from build123d import *

# Parameters (mm, degrees)
MODEL_R                  = 1.8
RESSALTO_EXTRUS_O1_DEPTH = 6


with BuildPart() as part:
    # Model → Ressalto-extrusão1 (new body)
    with BuildSketch(Plane.XY):
        Polygon((65.723755116, 35.074422304), (65.623854693, 35.315603259), (65.46493607, 35.52271004), (65.257829289, 35.681628662), (65.016648334, 35.781529085), (64.757829289, 35.815603259), (50.157829289, 35.815603259), (50.157829289, 33.103327835), (43.557829289, 33.103327835), (43.557829289, 56.603327835), (50.157829289, 56.603327835), (50.157829289, 50.820791423), (59.157829289, 50.820791423), (59.157829289, 56.103327835), (64.757829289, 56.103327835), (65.016648334, 56.137402008), (65.257829289, 56.237302431), (65.46493607, 56.396221053), (65.623854693, 56.603327835), (65.723755116, 56.844508789), (65.757829289, 57.103327835), (65.757829289, 61.703327835), (65.723755116, 61.96214688), (65.623854693, 62.203327835), (65.46493607, 62.410434616), (65.257829289, 62.569353238), (65.016648334, 62.669253661), (64.757829289, 62.703327835), (59.157829289, 62.703327835), (59.157829289, 67.703327835), (35.557829289, 67.703327835), (35.557829289, 59.703327835), (29.957829289, 59.703327835), (29.699010244, 59.669253661), (29.457829289, 59.569353238), (29.250722508, 59.410434616), (29.091803885, 59.203327835), (28.991903463, 58.96214688), (28.957829289, 58.703327835), (28.957829289, 50.703327835), (28.991903463, 50.444508789), (29.091803885, 50.203327835), (29.250722508, 49.996221053), (29.457829289, 49.837302431), (29.699010244, 49.737402008), (29.957829289, 49.703327835), (35.557829289, 49.703327835), (35.557829289, 30.703327835), (29.957829289, 30.703327835), (29.699010244, 30.669253661), (29.457829289, 30.569353238), (29.250722508, 30.410434616), (29.091803885, 30.203327835), (28.991903463, 29.96214688), (28.957829289, 29.703327835), (28.957829289, 21.703327835), (28.991903463, 21.444508789), (29.091803885, 21.203327835), (29.250722508, 20.996221053), (29.457829289, 20.837302431), (29.699010244, 20.737402008), (29.957829289, 20.703327835), (35.557829289, 20.703327835), (35.557829289, 12.703327835), (59.157829289, 12.703327835), (59.157829289, 20.903327835), (64.757829289, 20.903327835), (65.016648334, 20.937402008), (65.257829289, 21.037302431), (65.46493607, 21.196221053), (65.623854693, 21.403327835), (65.723755116, 21.644508789), (65.757829289, 21.903327835), (65.757829289, 34.815603259), align=None)
        with Locations((54.657829289, 63.703327835)):
            Circle(MODEL_R, mode=Mode.SUBTRACT)
        with Locations((54.657829289, 16.703327835)):
            Circle(MODEL_R, mode=Mode.SUBTRACT)
        Polygon((43.557829289, 23.803327835), (43.561764571, 18.803329383), (50.161762529, 18.808521259), (50.157829289, 23.808519712), align=None, mode=Mode.SUBTRACT)
        Polygon((50.557829289, 30.687927527), (50.557829289, 25.95365532), (54.657829289, 23.586519216), (58.757829289, 25.95365532), (58.757829289, 30.687927527), (54.657829289, 33.055063631), align=None, mode=Mode.SUBTRACT)
    extrude(amount=RESSALTO_EXTRUS_O1_DEPTH)


solid = part.part
Can you work these out from the model? Positions are in its coordinate system, mm. A direction names the side the tool comes from. Give positions to 0.01 mm unless a question says otherwise; leave off trailing zeros. Loops run counter-clockwise (first coordinate to the right, second up) from the corner with the lowest first, then second, coordinate; pieces in that order, holes last. Notation, with made-up numbers: (16.5, 22) - (49.5, 22) arc R17 ccw to (49.5, 39) - close; hole circle Ø2 at (86, 73). An arc over 180 degrees is marked (long way). Return JSON: item names as keys, results as strings.
1. If I drill on line 1 (Y direction, x = 44, z = 0.7); line 2 (X direction, y = 26.5, z = 4.15); line 3 (X direction, y = 16.5, z = 3.9), over which ranges is the centre line in solid material (lowest first)?
Output values:
{"line 1": "y = 12.7 to 18.8, 23.8 to 33.1, 56.6 to 67.7", "line 2": "x = 28.96 to 50.56, 58.76 to 65.76", "line 3": "x = 35.56 to 52.87, 56.45 to 59.16"}
2. I'm going to push flat-ended pins straight in: pin 1 Ø2 at (x, z) = (32.5, 1.5) entering from -Y; pin 2 Ø3 at (x, y) = (33.5, 45) entering from -Z; pin 3 Ø2.5 at (y, z) = (64.5, 4) entering from +X; pin 4 Ø1.5 at (y, z) = (62, 3.5) entering from -X. Where does each tip first touch, or does it pass through?
Output values:
{"pin 1": "stops at y = 20.7", "pin 2": "passes through", "pin 3": "stops at x = 59.16", "pin 4": "stops at x = 35.56"}
3. I want a section at D-D on x = 45. Please give me the cut outline in (y, z).
Output values:
{"outline": "(12.7, 0) - (18.8, 0) - (18.8, 6) - (12.7, 6) - close; (23.8, 0) - (33.1, 0) - (33.1, 6) - (23.8, 6) - close; (56.6, 0) - (67.7, 0) - (67.7, 6) - (56.6, 6) - close"}
4. I want a section at C-C on x = 53.5. Please give me the cut outline in (y, z) (3 decimals), and give its area (3 significant figures).
Output values:
{"outline": "(12.703, 0) - (15.325, 0) - (15.325, 6) - (12.703, 6) - close; (18.082, 0) - (24.255, 0) - (24.255, 6) - (18.082, 6) - close; (32.387, 0) - (35.816, 0) - (35.816, 6) - (32.387, 6) - close; (50.821, 0) - (62.325, 0) - (62.325, 6) - (50.821, 6) - close; (65.082, 0) - (67.703, 0) - (67.703, 6) - (65.082, 6) - close", "area": "158 mm²"}
5. I want a section at A-A on x = 34. Please give me the cut outline in (y, z), and give its area (3 significant figures).
Output values:
{"outline": "(20.7, 0) - (30.7, 0) - (30.7, 6) - (20.7, 6) - close; (49.7, 0) - (59.7, 0) - (59.7, 6) - (49.7, 6) - close", "area": "120 mm²"}
6. I want a section at B-B on y = 52.5. Please give me the cut outline in (x, z).
Output values:
{"outline": "(28.96, 0) - (43.56, 0) - (43.56, 6) - (28.96, 6) - close; (50.16, 0) - (59.16, 0) - (59.16, 6) - (50.16, 6) - close"}
7. For faces 1 (the face through (33, 30.703, 3)), 2 (the face through (52.64, 31.89, 2.96)), 3 (the face through (35.558, 64, 3)), which set-ups out of +Z, -Z, +X, -X, +Y, -Y let a thin tool reach every point of the face, with its end or its side?
Output values:
{"face 1": "+Z, -Z, -X", "face 2": "+Z, -Z", "face 3": "+Z, -Z, -X, +Y"}
8. We'd pull the mould along Y, two halves only. Please class faces 4 (the face through (59.158, 53, 3)), 5 (the face through (35.558, 17, 3)), 6 (the face through (33, 20.703, 3)): +Y half, -Y half, draft (parallel to the pull), parting line (faces both ways), or undercut.
Output values:
{"face 4": "undercut", "face 5": "draft", "face 6": "-Y half"}
